Answer from the drawing. Dimensions are ordinates in mm from the lowest x, y and z of the part. Coordinates: 2 decimals unless noted, no trailing zeros. Write each loop counter-clockwise with the first axis right and the second up, starting at its lowest first coordinate (ties: lowest second). Pieces come first, ordered by that corner, then holes. Notation, with made-up numbers: (-11.5, 29.25) - (18.5, 29.25) arc R33 ccw to (18.5, 67.25) - close; hole circle Ø2 at (41, 7.5). An arc over 180 degrees is marked (long way). Answer as a JSON object with one key per item and string values. Group by question number.
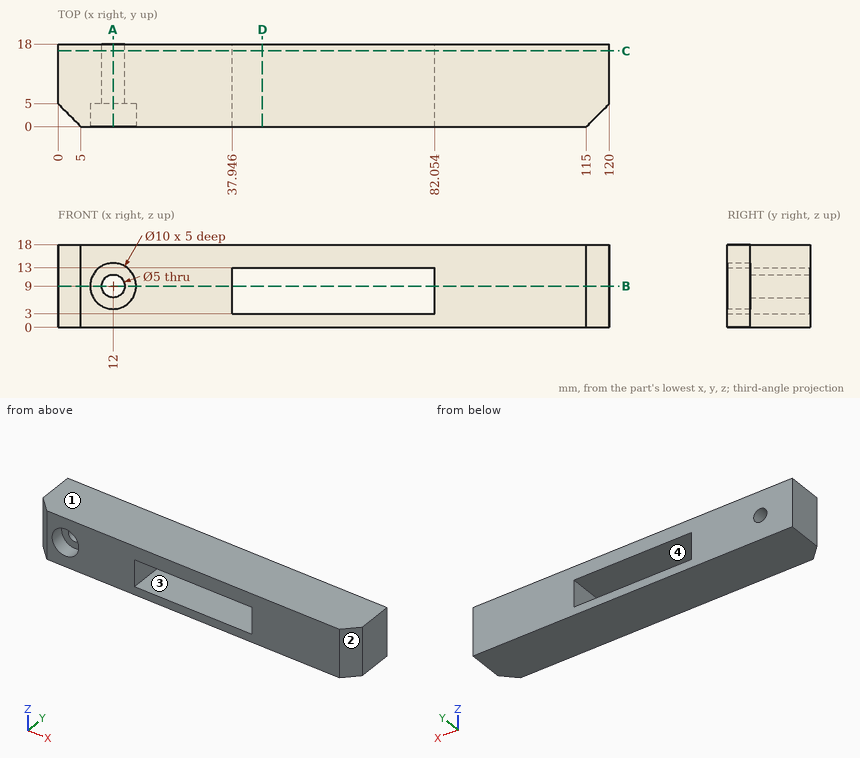
Q1. Flat-ended cylindrical pins translate along their axes: pin 1 Ø8 at (x, z) = (14, 7) entering from -Y; pin 2 Ø1 at (y, z) = (4, 2) entering from -X. Find the tip coordinate at first contact, or state that the pin passes through.
Q2. For a pull along Z with two mould halves and no side action, classify the marked faces 1, 2, 3 and 4 as +Z half, -Z half, draft (parallel to the pull), parting line (faces both ways), or undercut.
Q3. Section B-B on z = 9 is taken. Determine the outline of the cut face in (x, y) (1 decimal).
Q4. Section A-A on x = 12 is taken. Determine the outline of the cut face in (y, z).
Q5. Consider L1, parallel to X at y = 13, z = 8.75 (1 decimal); L2, parallel to Z at x = 12, y = 9.25; L3, parallel to Z at x = 12, y = 3.95. Determine where each line is inside the solid, lowest interval first. Write a range as from..to.
Q6. Section D-D on x = 44.5 is taken. Determine the outline of the cut face in (y, z).
Q7. Section C-C on y = 16.5 is taken. Determine the outline of the cut face in (x, z) (1 decimal), plus the area to 3 significant figures.
Numbers:
{
 "1": {"pin 1": "stops at y = 0", "pin 2": "stops at x = 0.5"},
 "2": {"face 1": "+Z half", "face 2": "draft", "face 3": "undercut", "face 4": "undercut"},
 "3": {"outline": "(0, 5) - (5, 0) - (7, 0) - (7, 5) - (9.5, 5) - (9.5, 18) - (0, 18) - close; (14.5, 5) - (17, 5) - (17, 0) - (37.9, 0) - (37.9, 18) - (14.5, 18) - close; (82.1, 0) - (115, 0) - (120, 5) - (120, 18) - (82.1, 18) - close"},
 "4": {"outline": "(0, 0) - (18, 0) - (18, 6.5) - (5, 6.5) - (5, 4) - (0, 4) - close; (0, 14) - (5, 14) - (5, 11.5) - (18, 11.5) - (18, 18) - (0, 18) - close"},
 "5": {"L1": "x = 0..9.5, 14.5..37.9, 82.1..120", "L2": "z = 0..6.5, 11.5..18", "L3": "z = 0..4, 14..18"},
 "6": {"outline": "(0, 0) - (18, 0) - (18, 3) - (0, 3) - close; (0, 13) - (18, 13) - (18, 18) - (0, 18) - close"},
 "7": {"outline": "(0, 0) - (120, 0) - (120, 18) - (0, 18) - close; hole circle Ø5 at (12, 9); hole (37.9, 3) - (82.1, 3) - (82.1, 13) - (37.9, 13) - close", "area": "1,700 mm²"}
}
